from build123d import *

# Parameters (mm, degrees)
F0_R     = 10
F0_R_2   = 1.5
F1_DEPTH = 1


with BuildPart() as f1:
    # F0 (on Front) → F1 (new body, symmetric)
    with BuildSketch(Plane.XZ):
        Circle(F0_R)
        with BuildLine():
            ThreePointArc((-2.514889, -2.592907), (-2.011909, -2.457202), (-1.508927, -2.592901))
            ThreePointArc((-1.508927, -2.592901), (0, -3), (1.508927, -2.592901))
            ThreePointArc((1.508927, -2.592901), (2.011909, -2.457202), (2.514889, -2.592907))
            Line((2.514889, -2.592907), (4.405493, -3.693166))
            ThreePointArc((4.405493, -3.693166), (4.89841, -4.467042), (4.552924, -5.317037))
            ThreePointArc((4.552924, -5.317037), (0, -7), (-4.552924, -5.317037))
            ThreePointArc((-4.552924, -5.317037), (-4.89841, -4.467042), (-4.405493, -3.693166))
            Line((-4.405493, -3.693166), (-2.514889, -2.592907))
        make_face(mode=Mode.SUBTRACT)
        with BuildLine():
            ThreePointArc((-6.881151, -1.28443), (-6.062178, 3.5), (-2.328227, 6.601466))
            ThreePointArc((-2.328227, 6.601466), (-1.419367, 6.475669), (-0.995629, 5.661851))
            Line((-0.995629, 5.661851), (-0.988079, 3.474412))
            ThreePointArc((-0.988079, 3.474412), (-1.122045, 2.970966), (-1.491055, 2.60322))
            ThreePointArc((-1.491055, 2.60322), (-2.598076, 1.5), (-2.999982, -0.010319))
            ThreePointArc((-2.999982, -0.010319), (-3.133954, -0.513764), (-3.502968, -0.881504))
            Line((-3.502968, -0.881504), (-5.401122, -1.968686))
            ThreePointArc((-5.401122, -1.968686), (-6.317777, -2.008627), (-6.881151, -1.28443))
        make_face(mode=Mode.SUBTRACT)
        Circle(F0_R_2, mode=Mode.SUBTRACT)
        with BuildLine():
            ThreePointArc((1.491055, 2.60322), (1.122045, 2.970966), (0.988079, 3.474412))
            Line((0.988079, 3.474412), (0.995629, 5.661851))
            ThreePointArc((0.995629, 5.661851), (1.419367, 6.475669), (2.328227, 6.601466))
            ThreePointArc((2.328227, 6.601466), (6.062178, 3.5), (6.881151, -1.28443))
            ThreePointArc((6.881151, -1.28443), (6.317777, -2.008627), (5.401122, -1.968686))
            Line((5.401122, -1.968686), (3.502968, -0.881504))
            ThreePointArc((3.502968, -0.881504), (3.133954, -0.513764), (2.999982, -0.010319))
            ThreePointArc((2.999982, -0.010319), (2.598076, 1.5), (1.491055, 2.60322))
        make_face(mode=Mode.SUBTRACT)
    extrude(amount=F1_DEPTH, both=True)

    # F2 (on Right) → F3 (revolve, cut)
    with BuildSketch(Plane.YZ):
        Polygon((0.75, 10), (0, 10), (0, 8.5), align=None)
        Polygon((0, 8.5), (0, 10), (-0.75, 10), align=None)
    revolve(axis=Axis((0, -0.179222, 0), (0, -1, 0)), mode=Mode.SUBTRACT)


solid = f1.part
Design review of the part built by this model. Coordinates are the model's own, in mm. A direction names the side the tool comes from. Coordinates: 2 decimals unless noted, no trailing zeros. Order: outer loops, then holes, each group sorted by start corner. A loop starts at its lowest first (then second) coordinate and runs counter-clockwise, first axis right, second up. Notation, with made-up numbers: M -21,-3 L 24,-3 A17 cw 24,20 Z; hole C 64.5,-38.75 d1. An arc over 180 degrees is marked long. Use a Markdown table: item, result.
(1) Add section A-A (x = 0). Give the boundary of the cut face in (y, z).
Worked answers:
| item | result |
|---|---|
| outline | M -1,-10 L -0.75,-10 L 0,-8.5 L 0.75,-10 L 1,-10 L 1,-7 L -1,-7 Z; M -1,-3 L 1,-3 L 1,-1.5 L -1,-1.5 Z; M -1,1.5 L 1,1.5 L 1,10 L 0.75,10 L 0,8.5 L -0.75,10 L -1,10 Z |
(2) Wall thickness on probe 1 along Z at (x, y) = (0, 0.4); probe 2 along X at (y, z) = (-0.6, 1); probe 3 along Z at (x, y) = (-4, -0.7): over which ranges is each line inside the solid? List them lowest first.
Worked answers:
| item | result |
|---|---|
| probe 1 | z = -9.3 to -7, -3 to -1.5, 1.5 to 9.3 |
| probe 2 | x = -9.65 to -6.93, -2.83 to -1.12, 1.12 to 2.83, 6.93 to 9.65 |
| probe 3 | z = -9.06 to -5.74, -3.46 to -1.17, 5.74 to 9.06 |
(3) For faces 1 (the cylindrical face through (-6.31, -0.01, -2.01)), 2 (the flat face through (2, -1, 0)), list the 3-axis set-ups (+Z, -Z, +X, -X, +Y, -Y) from which the entire face can be reached by the end or side of a thin tool; tool diameter is ignored.
Worked answers:
| item | result |
|---|---|
| face 1 | +Y, -Y |
| face 2 | +Z, -Z, +X, -X, -Y |
(4) Draft analysis for pull direction Z (two halves, no side actions). For faces 3 (the flat face through (2, 1, 0)), 4 (the cylindrical face through (-3.13, -0.01, -0.51)), state which applies: released by +Z, released by -Z, zero draft, split by the parting line, or undercut.
Worked answers:
| item | result |
|---|---|
| face 3 | zero draft |
| face 4 | undercut |
(5) Add section B-B (y = -0.25). Give the boundary of the cut face in (x, z), then the cut area to 3 significant figures.
Worked answers:
| item | result |
|---|---|
| outline | C 0,0 d18; hole M -6.88,-1.28 A1 ccw -5.4,-1.97 L -3.5,-0.88 A1 ccw -3,-0.01 A3 cw -1.49,2.6 A1 ccw -0.99,3.47 L -1,5.66 A1 ccw -2.33,6.6 A7 ccw Z; hole M -4.55,-5.32 A7 ccw 4.55,-5.32 A1 ccw 4.41,-3.69 L 2.51,-2.59 A1 ccw 1.51,-2.59 A3 cw -1.51,-2.59 A1 ccw -2.51,-2.59 L -4.41,-3.69 A1 ccw Z; hole C 0,0 d3; hole M 0.99,3.47 A1 ccw 1.49,2.6 A3 cw 3,-0.01 A1 ccw 3.5,-0.88 L 5.4,-1.97 A1 ccw 6.88,-1.28 A7 ccw 2.33,6.6 A1 ccw 1,5.66 Z |
| area | 148 mm2 |
(6) Add section C-C (z = 0.25). Count the separate pieces of the cut face and the enclosed holes in it, then the cut area to 3 significant figures.
Worked answers:
| item | result |
|---|---|
| separate pieces | 4 |
| enclosed holes | 0 |
| area | 15.8 mm2 |
